Autodesk Inventor part; units mm, degrees
ref_plane "Arbeitsebene1" through (45, 116.619, 0) normal (1, 0, 0) x (0, 0, -1)
ref_plane "YZ Plane" through (0, 0, 0) normal (1, 0, 0) x (0, 1, 0)
ref_plane "XZ Plane" through (0, 0, 0) normal (0, 1, 0) x (-1, 0, 0)
sketch "Skizze1" plane through (0, 0, 0) normal (0, 0, 1) x (1, 0, 0)
  arc A0 (-1.5, 4.7697) -> (1.5, 4.7697) centre (0, 0) ccw
  circle A1 centre (0, 0) radius 12.5
  line L0 (-30.9429, 0) -> (77.0229, 0) construction
  circle A2 centre (0, 0) radius 12.5
  circle A3 centre (45, 116.619) radius 16
  line L1 (61, 116.619) -> (61, 166.619)
  line L2 (29, 116.619) -> (29, 166.619)
  line L3 (45, 116.619) -> (45, 182.619) construction
  line L4 (45, 116.619) -> (45, 132.619) construction
  line L5 (29, 116.619) -> (61, 116.619) construction
  line L6 (-12.5, 0) -> (-12.5, 38.6768)
  line L7 (12.5, 0) -> (12.5, 38.6768)
  line L8 (-12.5, 38.6768) -> (12.5, 38.6768) construction
  circle A4 centre (0, 38.6768) radius 12.5 construction
  line L9 (-10.9271, 44.7471) -> (29, 116.619)
  arc A5 (-10.9271, 44.7471) -> (-12.5, 38.6768) centre (0, 38.6768) ccw
  line L10 (12.5, 38.6768) -> (58.3334, 107.7748)
  arc A6 (58.3334, 107.7748) -> (61, 116.619) centre (45, 116.619) ccw
  line L11 (0, 38.6768) -> (45, 116.619) construction
  circle A7 centre (45, 166.619) radius 16
  circle A8 centre (45, 166.619) radius 9.5
  circle A9 centre (45, 116.619) radius 9.5
  line L12 (-1.5, 6.4) -> (1.5, 6.4)
  line L13 (1.5, 6.4) -> (1.5, 4.7697)
  line L14 (-1.5, 4.7697) -> (-1.5, 6.4)
  line L15 (0, 0) -> (0, 5) construction
  line L16 (0, 5) -> (1.5, 5) construction
  circle A10 centre (45, 116.619) radius 12.75 construction
  circle A11 centre (45, 166.619) radius 12.75 construction
  circle A12 centre (45, 116.619) radius 10.5
  circle A13 centre (45, 166.619) radius 10.5
  circle A14 centre (45, 116.619) radius 12
  circle A15 centre (45, 166.619) radius 12
  point P0 (22.5, 77.6479)
  point P1 (45, 141.619)
  point P2 (0, 6.4)
  point P3 (45, 129.369)
  point P4 (33.9582, 110.244)
  point P5 (56.0418, 110.244)
  point P6 (45, 179.369)
  point P7 (33.9582, 160.244)
  point P8 (56.0418, 160.244)
  dimension "d69" = 25.5
  dimension "ParallelHebel_Passflansch_HoleDia" = 25.5
  dimension "d0" = 10
  dimension "d1" = 25
  dimension "d4" = 25
  dimension "d36" = 0
  dimension "ParallelHebel_Gabelgelenk_OuterDia" = 32
  dimension "d38" = 60
  dimension "d40" = 90
  dimension "d41" = 50
  dimension "d42" = 45
  dimension "d43" = 19
  dimension "Nadellager_OuterDia" = 19
  dimension "d45" = 25
  dimension "d51" = 3
  dimension "d52" = 1.4
  dimension "d67" = 360
  dimension "d72" = 360
  dimension "d83" = 21
  dimension "d84" = 24
  dimension "d85" = 21
  dimension "d86" = 24
  dimension "d91" = 125
extrude "Extrusion1" add sketch "Skizze1" along normal blind 6 contours A1
extrude "Extrusion2" add sketch "Skizze1" against normal blind 8 contours A1 | A1 L6 A5 L9 A3 L10 L7 | A3 | L2 A7 L1 A3 | A7 | A12 | A13 | A14 | A15
fillet "Rundung1" radius 25 2 edges at (29, 116.619, -4) (12.5, 38.6768, -4)
hole "Bohrung2" at (45, 141.619, 0) at (22.5, 77.6479, 0) direction (0, 0, -1) diameter 8 end through all
ref_plane "Arbeitsebene1" through (45, 116.619, 0) normal (1, 0, 0) x (0, 0, -1)
extrude "Extrusion5" cut sketch "Skizze1" against normal blind 1 contours A12 | A13 | A14 | A15
extrude "Extrusion6" cut sketch "Skizze1" against normal blind 1 from surface at -1 contours A12 | A13
equation "\"d1_1\" = 25"
equation "\"d8_1\" = 0"
equation "\"d10_1\" = 0"
equation "\"d11_1\" = 25"
equation "\"d23_1\" = 8"
equation "\"d36_1\" = 0"
equation "\"d38_1\" = 60deg"
equation "\"d39_1\" = 35"
equation "\"ParallelLink_Lever_Thickness_1\" = 14"
equation "\"ParallelHebel_Gabelgelenk_OuterDia_1\" = 32"
equation "\"Nadellager_OuterDia_1\" = 19"
equation "\"ParallelHebel_Passflansch_HoleDia_1\" = 25.5"
equation "\"d1_1_2_3\" = 25"
equation "\"ParallelMecha_Bearing_Step_Thickness\" = 6"
equation "\"d8_1_2_3\" = 0"
equation "\"d39_1_2\" = 35"
properties part number "ParallelSystem_ProximalPart_Driven_Counterpart_v2.1_Rillenkugellager" material "Aluminium 6061"
For this review, take the finished solid that the model builds, in its own axes (mm). A direction names the side the tool comes from. Give positions to 0.01 mm unless a question says otherwise; leave off trailing zeros. Write each loop counter-clockwise with the first axis right and the second up, starting at its lowest first coordinate (ties: lowest second). Pieces come first, ordered by that corner, then holes. Notation, with made-up numbers: M -16,77 L 38,77 A21 ccw 38,105 Z; hole C -3.75,-15 d4. An arc over 180 degrees is marked long. One line per item, written item: value.
1) For line 1 (Y direction, x = 45, z = -0.2); line 2 (Y direction, x = 45, z = -1.3); line 3 (Z direction, x = 29.5, y = 110), list the stretches that pass through material, from the lowest coordinate up. Write a range as from..to.
Results are:
line 1: y = 87.67..104.62, 128.62..137.62, 145.62..154.62, 178.62..182.62
line 2: y = 87.67..106.12, 127.12..137.62, 145.62..156.12, 177.12..182.62
line 3: z = -8..0
2) The part is to be moulded in two halves that separate along Y. For faces 1 (the flat face through (21, 92, 0)), 2 (the cylindrical face through (13.535, 38.258, -4.056)), 3 (the flat face through (46, 156, -1)), 4 (the flat face through (37, 161, -2)), say which applies: +Y half, -Y half, draft (parallel to the pull), parting line (faces both ways), or undercut.
Results are:
face 1: draft
face 2: -Y half
face 3: undercut
face 4: undercut
3) For faces 5 (the flat face through (29, 145, -4)), 6 (the flat face through (24, 86, -8)), 7 (the cylindrical face through (34.51, 117.08, -1.49)), list the 3-axis set-ups (+Z, -Z, +X, -X, +Y, -Y) from which the entire face can be reached by the end or side of a thin tool; tool diameter is ignored.
Results are:
face 5: +Z, -Z, -X, +Y
face 6: -Z, +X, -X, +Y, -Y
face 7: +Z
4) Take a section at C-C, the plane y = 140. Write out the cut boundary in (x, z), then the cut area to 3 significant figures.
Results are:
outline: M 29,-8 L 41.34,-8 L 41.34,0 L 29,0 Z; M 48.66,-8 L 61,-8 L 61,0 L 48.66,0 Z
area: 197 mm²
5) Take a section at B-B, the plane x = 38. Write out the cut boundary in (y, z), then the cut area to 3 significant figures.
Results are:
outline: M 77.12,-8 L 110.2,-8 L 110.2,-2 L 108.79,-2 L 108.79,-1 L 106.87,-1 L 106.87,0 L 77.12,0 Z; M 123.04,-8 L 160.2,-8 L 160.2,-2 L 158.79,-2 L 158.79,-1 L 156.87,-1 L 156.87,0 L 126.37,0 L 126.37,-1 L 124.45,-1 L 124.45,-2 L 123.04,-2 Z; M 173.04,-8 L 181.01,-8 L 181.01,0 L 176.37,0 L 176.37,-1 L 174.45,-1 L 174.45,-2 L 173.04,-2 Z
area: 607 mm²
6) Take a section at D-D, the plane x = 20.5. Write out the cut boundary in (y, z).
Results are:
outline: M 50.74,-8 L 74.18,-8 L 74.18,0 L 50.74,0 Z; M 81.11,-8 L 101.32,-8 L 101.32,0 L 81.11,0 Z
7) Take a section at A-A, the plane z = 1.75. Write out the cut boundary in (x, y), then the cut area to 3 significant figures.
Results are:
outline: C 0,0 d25; hole M -1.5,4.77 A5 ccw long 1.5,4.77 L 1.5,6.4 L -1.5,6.4 Z
area: 408 mm²
8) For P1, Ø4, axis at y = 150.5, z = -4.5, coming from the -X side; P2, Ø0.8, axis at y = 5.5, z = 2, coming from the +X side; P3, Ø17, axis at x = 40.5, y = 168.5, coming from the +Z side; P4, Ø8, axis at x = 47.5, y = 117.5, coming from the -Z side, all flat-tipped, find the tip position at first contact; note any pin that passes through.
Results are:
P1: stops at x = 29
P2: stops at x = 11.41
P3: stops at z = 0
P4: passes through
